Drawing for the job (mm, zero at the part's lowest x, y, z). Give positions to 0.01 mm unless a question says otherwise; leave off trailing zeros. Write each loop counter-clockwise with the first axis right and the second up, starting at its lowest first coordinate (ties: lowest second). Pieces come first, ordered by that corner, then holes. Notation, with made-up numbers: M 50.5,-5.5 L 109.5,-5.5 A12 cw 109.5,5.5 Z; hole C 18.25,31 d9. An arc over 180 degrees is marked long. Answer as a JSON object with one key per item and string values. Group by question number.
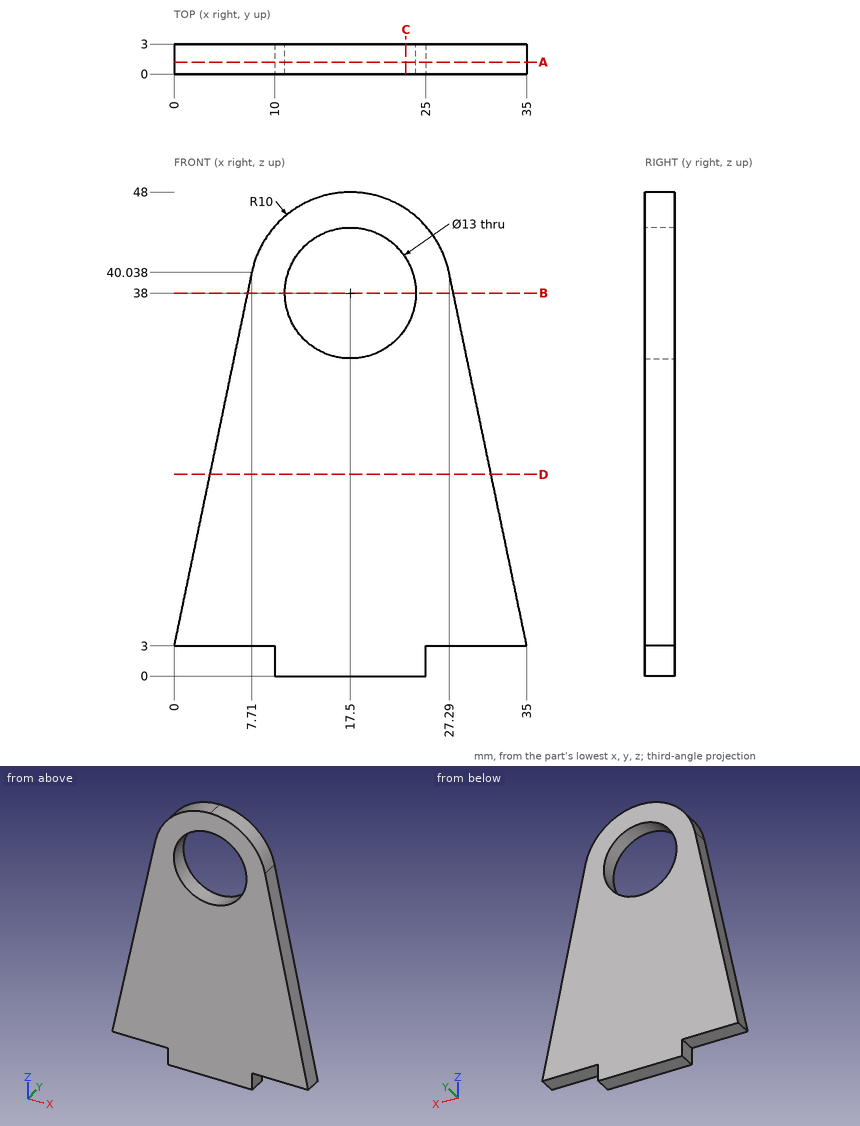
Q1. Wall check: L1, parallel to X at y = 2.85, z = 38; L2, parallel to X at y = 1.6, z = 32; L3, parallel to Z at x = 26.5, y = 2.85. Give the ranges that are in metal, low to high.
Q2. Drop flat-ended pins along their axis: P1, Ø11.5, axis at x = 17.5, z = 38, coming from the -Y side; P2, Ø1, axis at y = 2.5, z = 7, coming from the +X side; P3, Ø1.5, axis at x = 5, y = 1, coming from the -Z side. Give the stop position or say it passes through.
Q3. Slice it at D-D, the plane z = 20. Write the cut outline in (x, y).
Q4. Slice it at B-B, the plane z = 38. Write the cut outline in (x, y), then the cut area to 3 significant figures.
Q5. Slice it at A-A, the plane y = 1.2. Write the cut outline in (x, z).
Q6. Slice it at C-C, the plane x = 23. Write the cut outline in (y, z).
Solved:
{
 "1": {"L1": "x = 7.29 to 11, 24 to 27.71", "L2": "x = 6.04 to 15, 20 to 28.96", "L3": "z = 3 to 42.36"},
 "2": {"P1": "passes through", "P2": "stops at x = 34.27", "P3": "stops at z = 3"},
 "3": {"outline": "M 3.54,0 L 31.46,0 L 31.46,3 L 3.54,3 Z"},
 "4": {"outline": "M 7.29,0 L 11,0 L 11,3 L 7.29,3 Z; M 24,0 L 27.71,0 L 27.71,3 L 24,3 Z", "area": "22.3 mm²"},
 "5": {"outline": "M 0,3 L 10,3 L 10,0 L 25,0 L 25,3 L 35,3 L 27.29,40.04 A10 ccw 17.5,48 A10 ccw 7.71,40.04 Z; hole C 17.5,38 d13"},
 "6": {"outline": "M 0,0 L 3,0 L 3,34.54 L 0,34.54 Z; M 0,41.46 L 3,41.46 L 3,46.35 L 0,46.35 Z"}
}
